Autodesk Inventor part; units mm, degrees
ref_plane "YZ Plane" through (0, 0, 0) normal (1, 0, 0) x (0, 1, 0)
ref_plane "XZ Plane" through (0, 0, 0) normal (0, 1, 0) x (-1, 0, 0)
ref_plane "XY Plane" through (0, 0, 0) normal (0, 0, 1) x (1, 0, 0)
sketch "Sketch1" plane through (0, 0, 0) normal (0, 0, 1) x (1, 0, 0)
  line L0 (0, 0) -> (122, 0)
  circle A0 centre (61, 52) radius 45
  line L1 (3, 78.943) -> (20, 78.943)
  line L2 (20, 78.943) -> (42, 102)
  line L3 (42, 102) -> (80, 102)
  line L4 (80, 102) -> (102, 78.943)
  line L5 (102, 78.943) -> (119, 78.943)
  line L6 (3, 25.057) -> (0, 22.057)
  line L7 (0, 22.057) -> (0, 0)
  line L8 (122, 0) -> (122, 22.057)
  line L9 (122, 22.057) -> (119, 25.057)
  line L10 (119, 25.057) -> (119, 78.943)
  line L11 (16, 52) -> (3, 52)
  line L12 (3, 52) -> (3, 25.057)
  line L13 (3, 52) -> (3, 78.943)
  point P0 (61, 0)
  point P1 (61, 102)
  dimension "d3" = 90
  dimension "d0" = 79
  dimension "d1" = 122
  dimension "d2" = 52
  dimension "d4" = 17
  dimension "d5" = 38
  dimension "d6" = 102
  dimension "d7" = 116
  dimension "d8" = 135
extrude "Extrusion1" add sketch "Sketch1" along normal blind 72
sketch "Sketch2" plane through (0, 0, 0) normal (0, -1, 0) x (1, 0, 0)
  line L0 (11, 11) -> (111, 11) construction
  line L1 (111, 11) -> (111, 61) construction
  line L2 (111, 61) -> (11, 61) construction
  line L3 (11, 61) -> (11, 11) construction
  circle A0 centre (11, 11) radius 4.5
  circle A1 centre (111, 11) radius 4.5
  circle A2 centre (111, 61) radius 4.5
  circle A3 centre (11, 61) radius 4.5
  line L4 (0, 72) -> (122, 72) construction
  line L5 (0, 0) -> (0, 72) construction
  point P0 (61, 61)
  point P1 (61, 72)
  point P2 (11, 36)
  point P3 (0, 36)
  dimension "d11" = 100
  dimension "d12" = 50
  dimension "d13" = 9
extrude "Extrusion2" cut sketch "Sketch2" against normal up to surface (78.943 mm away)
properties part number "Spindle_Holder"
For this review, take the finished solid that the model builds, in its own axes (mm). A direction names the side the tool comes from. Round coordinates to 2 decimals unless told otherwise and drop trailing zeros. Order: outer loops, then holes, each group sorted by start corner. A loop starts at its lowest first (then second) coordinate and runs counter-clockwise, first axis right, second up.
Q1. We need section D-D, the plane z = 21.5. Give the boundary of the cut face in (x, y).
Findings below:
outline: (0, 0) - (122, 0) - (122, 22.06) - (119, 25.06) - (119, 78.94) - (102, 78.94) - (80, 102) - (42, 102) - (20, 78.94) - (3, 78.94) - (3, 25.06) - (0, 22.06) - close; hole circle Ø90 at (61, 52)
Q2. Wall thickness on line 1 (Z direction, x = 11, y = 26); line 2 (X direction, y = 52, z = 24); line 3 (Z direction, x = 8.5, y = 7.5): over which ranges is each line inside the solid? List them lowest first.
Findings below:
line 1: z = 0 to 6.5, 15.5 to 56.5, 65.5 to 72
line 2: x = 3 to 16, 106 to 119
line 3: z = 0 to 7.26, 14.74 to 57.26, 64.74 to 72
Q3. Machinability: for faces 4 (the flat face through (60, 0, 35)), 5 (the flat face through (119, 52, 35)), 6 (the flat face through (3, 52, 35)), which of the approach directions +Z, -Z, +X, -X, +Y, -Y give a long, thin tool a straight path to every point of the face, cutting with its end or side? Answer none if there is none.
Findings below:
face 4: +Z, -Z, +X, -X, -Y
face 5: +Z, -Z, +X, +Y
face 6: +Z, -Z, -X, +Y
Q4. We need section A-A, the plane y = 52. Give the boundary of the cut face in (x, z), plus the area to 3 significant figures.
Findings below:
outline: (3, 0) - (16, 0) - (16, 72) - (3, 72) - close; (106, 0) - (119, 0) - (119, 72) - (106, 72) - close; hole circle Ø9 at (11, 11); hole circle Ø9 at (11, 61); hole circle Ø9 at (111, 11); hole circle Ø9 at (111, 61)
area: 1,620 mm2
Q5. Insertion check: P1, Ø8, axis at x = 111, z = 61, coming from the +Y side; P2, Ø18.5, axis at x = 15.5, z = 49, coming from the +Y side; P3, Ø5, axis at x = 109.5, z = 37, coming from the +Y side. Each pin has a flat end and moves straight along its axis. Give the tip position at first contact, or say it passes through.
Findings below:
P1: passes through
P2: stops at y = 83.92
P3: stops at y = 78.94
Q6. Mouldability with a two-part tool opening along Y and no side actions: class faces 1 (the cylindrical face through (25, 79, 35)), 2 (the flat face through (0, 11, 35)), 3 (the flat face through (110, 78.943, 35)) as pulls with the +Y half, pulls with the -Y half, needs draft (parallel to the pull), parting line crosses it, or undercut.
Findings below:
face 1: undercut
face 2: needs draft
face 3: pulls with the +Y half
Q7. We need section B-B, the plane z = 61. Give the boundary of the cut face in (x, y), plus the area to 3 significant figures.
Findings below:
outline: (0, 0) - (6.5, 0) - (6.5, 78.94) - (3, 78.94) - (3, 25.06) - (0, 22.06) - close; (15.5, 0) - (106.5, 0) - (106.5, 78.94) - (102, 78.94) - (80, 102) - (42, 102) - (20, 78.94) - (15.5, 78.94) - close; (115.5, 0) - (122, 0) - (122, 22.06) - (119, 25.06) - (119, 78.94) - (115.5, 78.94) - close; hole circle Ø90 at (61, 52)
area: 2,900 mm2
Q8. We need section C-C, the plane x = 111. Give the boundary of the cut face in (y, z), plus the area to 3 significant figures.
Findings below:
outline: (0, 0) - (78.94, 0) - (78.94, 6.5) - (0, 6.5) - close; (0, 15.5) - (78.94, 15.5) - (78.94, 56.5) - (0, 56.5) - close; (0, 65.5) - (78.94, 65.5) - (78.94, 72) - (0, 72) - close
area: 4,260 mm2
